from build123d import *

# Parameters (mm, degrees)
SKETCH2_W           = 9.65
SKETCH2_H           = 3.6
BOSS_EXTRUDE1_DEPTH = 15
SKETCH4_W           = 14
SKETCH4_H           = 7
CUT_EXTRUDE1_DEPTH  = 112.070154559
SKETCH5_W           = 13.5
SKETCH5_H           = 15
BOSS_EXTRUDE2_DEPTH = 1.2
SKETCH6_W           = 3
SKETCH6_H           = 0.5
BOSS_EXTRUDE3_DEPTH = 4
LPATTERN1_COUNT     = 4
LPATTERN1_PITCH     = 3
BOSS_EXTRUDE4_DEPTH = 4
FILLET1_R           = 0.5


with BuildPart() as part:
    # Sketch2 → Boss-Extrude1 (new body)
    with BuildSketch(Plane.XY):
        Polygon((-76.021288744, 76.276019576), (-76.021288744, 79.576019576), (-49.321288744, 79.576019576), (-49.321288744, 76.276019576), (-53.021288744, 76.276019576), (-53.021288744, 72.576019576), (-72.321288744, 72.576019576), (-72.321288744, 76.276019576), align=None)
        with Locations((-57.846288744, 70.776019576)):
            Rectangle(SKETCH2_W, SKETCH2_H)
        with Locations((-67.496288744, 70.776019576)):
            Rectangle(SKETCH2_W, SKETCH2_H)
    extrude(amount=BOSS_EXTRUDE1_DEPTH)

    # Sketch4 → Cut-Extrude1 (cut, through all)
    with BuildSketch(Plane(origin=(0, 0, 0), x_dir=(-1, 0, 0), z_dir=(0, 0, -1))):
        with Locations((62.671288744, 76.076019576)):
            Rectangle(SKETCH4_W, SKETCH4_H)
    extrude(amount=-CUT_EXTRUDE1_DEPTH, mode=Mode.SUBTRACT)

    # Sketch5 → Boss-Extrude2 (add)
    with BuildSketch(Plane(origin=(0, 79.576019576, 0), x_dir=(1, 0, 0), z_dir=(0, 1, 0))):
        with Locations((-62.921288744, -7.5)):
            Rectangle(SKETCH5_W, SKETCH5_H)
    extrude(amount=-BOSS_EXTRUDE2_DEPTH)

    # Sketch6 → Boss-Extrude3 (add)
    with BuildSketch(Plane(origin=(-56.171288744, 0, 0), x_dir=(0, 0, -1), z_dir=(1, 0, 0))):
        with Locations((-12, 79.826019576)):
            Rectangle(SKETCH6_W, SKETCH6_H)
        Polygon((-10.5, 80.076019576), (-13.5, 80.076019576), (-12, 81.576019576), align=None)
    boss_extrude3 = extrude(amount=-BOSS_EXTRUDE3_DEPTH)

    # LPattern1: Boss-Extrude3 ×4
    with Locations(*[(0, 0, -i * LPATTERN1_PITCH) for i in range(1, LPATTERN1_COUNT)]):
        add(boss_extrude3)

    # Sketch7 → Boss-Extrude4 (add)
    with BuildSketch(Plane(origin=(-56.171288744, 0, 0), x_dir=(0, 0, -1), z_dir=(1, 0, 0))):
        Polygon((-13.5, 80.076019576), (-13.5, 79.576019576), (-14, 79.576019576), align=None)
        Polygon((-1.5, 80.076019576), (-1.5, 79.576019576), (-1, 79.576019576), align=None)
    extrude(amount=-BOSS_EXTRUDE4_DEPTH)

    # Fillet1
    fillet1_edges = [part.edges().sort_by_distance(p)[0] for p in [
        (-76.021288744, 76.276019576, 7.5),
        (-76.021288744, 79.576019576, 7.5),
        (-76.021288744, 77.926019576, 0),
        (-76.021288744, 77.926019576, 15),
        (-74.171288744, 76.276019576, 15),
        (-66.096288744, 79.576019576, 15),
        (-62.921288744, 78.376019576, 15),
        (-69.671288744, 75.476019576, 15),
        (-62.671288744, 72.576019576, 15),
        (-55.671288744, 76.076019576, 15),
        (-49.321288744, 77.926019576, 15),
        (-51.171288744, 76.276019576, 15),
        (-53.021288744, 72.626019576, 15),
        (-62.671288744, 68.976019576, 15),
        (-72.321288744, 72.626019576, 15),
        (-72.321288744, 76.276019576, 7.5),
        (-72.321288744, 72.626019576, 0),
        (-72.321288744, 68.976019576, 7.5),
        (-53.021288744, 68.976019576, 7.5),
        (-62.671288744, 68.976019576, 0),
        (-53.021288744, 76.276019576, 7.5),
        (-53.021288744, 72.626019576, 0),
        (-49.321288744, 76.276019576, 7.5),
        (-51.171288744, 76.276019576, 0),
        (-49.321288744, 79.576019576, 7.5),
        (-49.321288744, 77.926019576, 0),
        (-55.671288744, 79.576019576, 7.5),
        (-55.671288744, 76.076019576, 0),
        (-55.671288744, 72.576019576, 7.5),
        (-62.671288744, 72.576019576, 0),
        (-69.671288744, 72.576019576, 7.5),
        (-69.671288744, 75.476019576, 0),
        (-69.671288744, 78.376019576, 7.5),
        (-62.921288744, 78.376019576, 0),
        (-56.171288744, 78.376019576, 7.5),
        (-56.171288744, 79.576019576, 14.5),
        (-56.171288744, 80.576019576, 13),
        (-56.171288744, 80.576019576, 2),
        (-56.171288744, 79.576019576, 0.5),
        (-58.171288744, 79.576019576, 1),
        (-58.171288744, 81.576019576, 3),
        (-60.171288744, 79.576019576, 7.5),
        (-58.171288744, 81.576019576, 6),
        (-58.171288744, 81.576019576, 9),
        (-58.171288744, 81.576019576, 12),
        (-58.171288744, 79.576019576, 14),
        (-74.171288744, 76.276019576, 0),
        (-66.096288744, 79.576019576, 0),
    ]]
    fillet(fillet1_edges, radius=FILLET1_R - 0.0001)  # a hair under: the kernel refuses the full size


solid = part.part
Can you work these out from the model? Positions are in its coordinate system, mm. A direction names the side the tool comes from. Give positions to 0.01 mm unless a question says otherwise; leave off trailing zeros. Write each loop counter-clockwise with the first axis right and the second up, starting at its lowest first coordinate (ties: lowest second). Pieces come first, ordered by that corner, then holes. Notation, with made-up numbers: (12.5, -27) -> (69.5, -27) arc R16 cw to (69.5, -18) -> close; hole circle Ø11 at (-14.75, 85). An arc over 180 degrees is marked (long way). Answer as a JSON object with one key per item and string values. Group by question number.
Item 1: Suppose I cut it at D-D (y = 71). Please give me the cut outline in (x, z).
Item 2: Please list where these lines run through material, in increasing order: line 1 (X direction, y = 75.5, z = 9.5); line 2 (Y direction, x = -63.75, z = 12.5); line 3 (Z direction, x = -60, y = 80.25). Write a range as [from, to].
Item 3: Suppose I cut it at B-B (y = 74.5). Please give me the cut outline in (x, z).
Item 4: We'd pull the mould along Z, two halves only. Please class faces 1 (the face through (-56.32, 80.56, 12.81)), 2 (the face through (-56.314, 80.556, 2.192)), 3 (the face through (-69.671, 75, 7)), 4 (the face through (-58.143, 80.641, 6.935)): +Z half, -Z half, draft (parallel to the pull), parting line (faces both ways), or undercut.
Item 5: For faces 5 (the face through (-53, 79.576, 7)), 6 (the face through (-53.021, 73, 7)), 7 (the face through (-56.171, 80, 7)), 8 (the face through (-63, 78.376, 7)), which set-ups out of +Z, -Z, +X, -X, +Y, -Y let a thin tool reach every point of the face, with its end or its side?
Item 6: I'm going to push flat-ended pins straight in: P1, Ø6, axis at x = -64, z = 13, coming from the +Y side; P2, Ø2, axis at y = 71, z = 6, coming from the +X side; P3, Ø1.2, axis at y = 80, z = 9.5, coming from the +X side. Where does each tip first touch, or does it pass through?
Findings:
{
 "1": {"outline": "(-72.32, 0.5) arc R0.5 ccw to (-71.82, 0) -> (-53.52, 0) arc R0.5 ccw to (-53.02, 0.5) -> (-53.02, 14.5) arc R0.5 ccw to (-53.52, 15) -> (-71.82, 15) arc R0.5 ccw to (-72.32, 14.5) -> close"},
 "2": {"line 1": "x = [-72.32, -69.67], [-55.67, -53.02]", "line 2": "y = [68.98, 72.58], [78.38, 79.58]", "line 3": "z = [1.67, 4.33], [4.67, 7.33], [7.67, 10.33], [10.67, 13.33]"},
 "3": {"outline": "(-72.32, 0.5) arc R0.5 ccw to (-71.82, 0) -> (-70.17, 0) arc R0.5 ccw to (-69.67, 0.5) -> (-69.67, 14.5) arc R0.5 ccw to (-70.17, 15) -> (-71.82, 15) arc R0.5 ccw to (-72.32, 14.5) -> close; (-55.67, 0.5) arc R0.5 ccw to (-55.17, 0) -> (-53.52, 0) arc R0.5 ccw to (-53.02, 0.5) -> (-53.02, 14.5) arc R0.5 ccw to (-53.52, 15) -> (-55.17, 15) arc R0.5 ccw to (-55.67, 14.5) -> close"},
 "4": {"face 1": "+Z half", "face 2": "-Z half", "face 3": "draft", "face 4": "undercut"},
 "5": {"face 5": "+Z, -Z, +X, +Y", "face 6": "+Z, -Z, +X, -Y", "face 7": "+Z, -Z, +Y", "face 8": "+Z, -Z"},
 "6": {"P1": "stops at y = 79.58", "P2": "stops at x = -53.02", "P3": "stops at x = -49.44"}
}
